Design review of the part shown in the three views and the two pictorial views. Dimensions are in mm from the part's minimum x, y and z. A direction names the side the tool comes from. Round coordinates to 2 decimals unless told otherwise and drop trailing zeros. Order: outer loops, then holes, each group sorted by start corner. A loop starts at its lowest first (then second) coordinate and runs counter-clockwise, first axis right, second up. Notation, with made-up numbers: (-31, 64.5) - (-4, 64.5) arc R20 cw to (-4, 73.5) - close; hole circle Ø7 at (28, 21.5). An arc over 180 degrees is marked (long way). One line per question, with ' | ' between items. Start each with the question number.
Item 1: Tool access review of the marked faces 5 and 6: name each direction out of +Z, -Z, +X, -X, +Y, -Y from which nothing blocks a thin tool from reaching the whole face with its end or side.
Item 2: Add section A-A on y = 51.5. State the section outline as (x, z) points.
Item 3: Add section B-B on x = 8. State the section outline as (y, z) points.
Item 4: Draft analysis for pull direction X (two halves, no side actions). For the marked faces 1, 2, 3 and 4, state which applies: +X half, -X half, draft (parallel to the pull), parting line (faces both ways), or undercut.
Item 5: Add section C-C on z = 6.75. State the section outline as (x, y) points, and give its area (3 significant figures).
Item 6: For L1, parallel to Y at x = 8, z = 3.75; L2, parallel to X at y = 27.5, z = 0.75; L3, parallel to X at y = 80, z = 5, list the stretches that pass through material, from the lowest coordinate up. Write a range as [from, to].
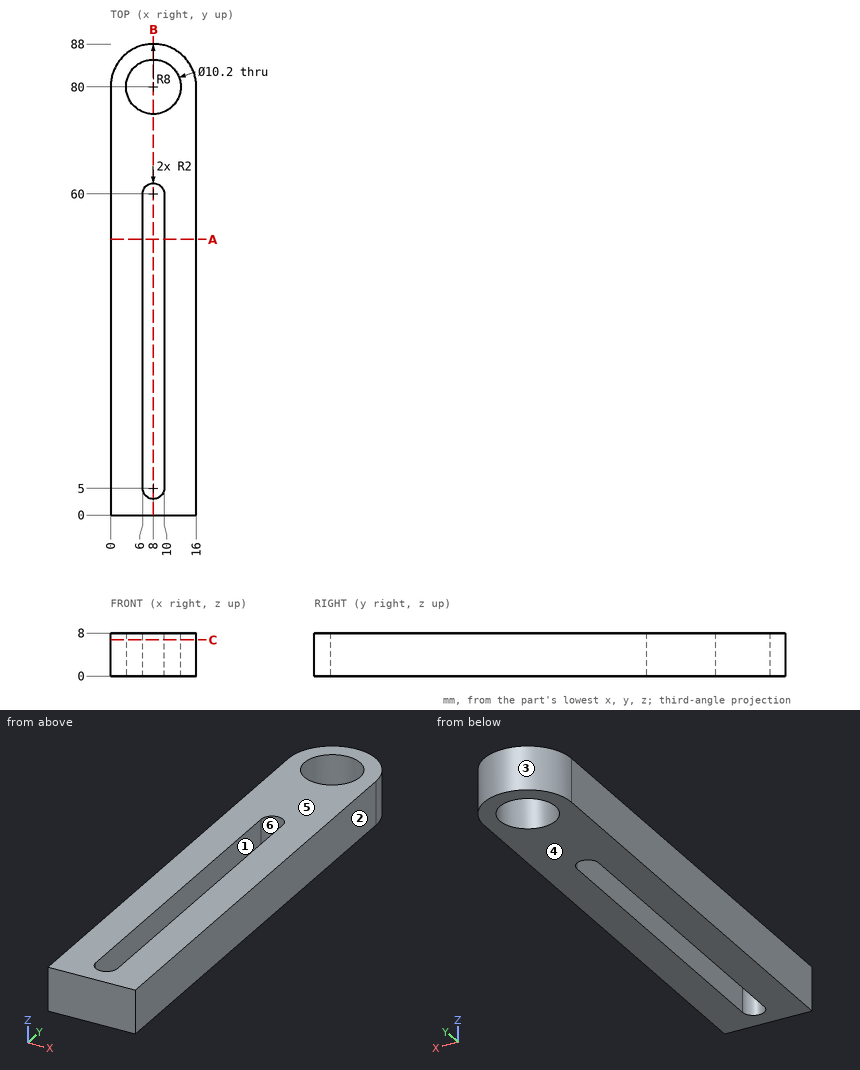
Determined:
1) face 5: +Z, +X, -X, +Y, -Y | face 6: +Z, -Z
2) outline: (0, 0) - (6, 0) - (6, 8) - (0, 8) - close; (10, 0) - (16, 0) - (16, 8) - (10, 8) - close
3) outline: (0, 0) - (3, 0) - (3, 8) - (0, 8) - close; (62, 0) - (74.9, 0) - (74.9, 8) - (62, 8) - close; (85.1, 0) - (88, 0) - (88, 8) - (85.1, 8) - close
4) face 1: undercut | face 2: +X half | face 3: parting line | face 4: draft
5) outline: (0, 0) - (16, 0) - (16, 80) arc R8 ccw to (0, 80) - close; hole circle Ø10.2 at (8, 80); hole (6, 5) arc R2 ccw to (10, 5) - (10, 60) arc R2 ccw to (6, 60) - close | area: 1,070 mm2
6) L1: [0, 3], [62, 74.9], [85.1, 88] | L2: [0, 6], [10, 16] | L3: [0, 2.9], [13.1, 16]
